```python
from build123d import *

# Parameters (mm, degrees)
CROQUIS2_W              = 20
CROQUIS2_H              = 10
SALIENTE_EXTRUIR1_DEPTH = 3
SALIENTE_EXTRUIR2_DEPTH = 2
CROQUIS4_W              = 3.2
CROQUIS4_H              = 5.473345926
CORTAR_EXTRUIR1_DEPTH   = 4
CROQUIS5_R              = 2.25
SALIENTE_EXTRUIR3_DEPTH = 3.2
CROQUIS6_R              = 1.5
CORTAR_EXTRUIR2_DEPTH   = 24.003733896
CROQUIS7_W              = 0.6
CROQUIS7_H              = 4.5
SALIENTE_EXTRUIR4_DEPTH = 1.75
CROQUIS8_R              = 0.9
CORTAR_EXTRUIR3_DEPTH   = 28.017462518


with BuildPart() as part:
    # Croquis2 → Saliente-Extruir1 (new, symmetric)
    with BuildSketch(Plane(origin=(0, 0, 0), x_dir=(0, 0, -1), z_dir=(1, 0, 0))):
        Rectangle(CROQUIS2_W, CROQUIS2_H)
    extrude(amount=SALIENTE_EXTRUIR1_DEPTH, both=True)

    # Croquis3 → Saliente-Extruir2 (add, symmetric)
    with BuildSketch(Plane(origin=(0, 0, 0), x_dir=(0, 0, -1), z_dir=(1, 0, 0))):
        with BuildLine():
            Line((-4.3, 5), (-4.3, 6.3))
            ThreePointArc((-4.3, 6.3), (-4.153553391, 6.653553391), (-3.8, 6.8))
            Line((-3.8, 6.8), (-2.5, 6.8))
            ThreePointArc((-2.5, 6.8), (-2.146446609, 6.653553391), (-2, 6.3))
            Line((-2, 6.3), (-2, 5))
            Line((-2, 5), (-4.3, 5))
        make_face()
        with BuildLine():
            Line((-7.25, 5), (-7.559492191, 6.592199292))
            Line((-7.559492191, 6.592199292), (6.919218672, 13.724276953))
            Line((6.919218672, 13.724276953), (5.46098718, 16.68460817))
            ThreePointArc((5.46098718, 16.68460817), (6.257555216, 19.027785364), (8.60073241, 18.231217328))
            Line((8.60073241, 18.231217328), (10.235719234, 14.912058085))
            Line((10.235719234, 14.912058085), (-6.654286119, 6.592199292))
            Line((-6.654286119, 6.592199292), (-7.115345765, 6.365085619))
            Line((-7.115345765, 6.365085619), (-6.85, 5))
            Line((-6.85, 5), (-7.25, 5))
        make_face()
    extrude(amount=SALIENTE_EXTRUIR2_DEPTH, both=True)

    # Croquis4 → Cortar-Extruir1 (cut)
    with BuildSketch(Plane(origin=(0, 5.422686469, -11.008504563), x_dir=(1, 0, 0), z_dir=(0, -0.4418883309364162, 0.8970700658155017))):
        with Locations((0, 11.990789002)):
            Rectangle(CROQUIS4_W, CROQUIS4_H)
    extrude(amount=-CORTAR_EXTRUIR1_DEPTH, mode=Mode.SUBTRACT)

    # Croquis5 → Saliente-Extruir3 (add)
    with BuildSketch(Plane.ZY.offset(-1.6)):
        with Locations(Location((-7.030859795, 17.457912749, 0), (0, 0, 192.71801499))):
            Circle(CROQUIS5_R)
    extrude(amount=SALIENTE_EXTRUIR3_DEPTH)

    # Croquis6 → Cortar-Extruir2 (cut, through all)
    with BuildSketch(Plane(origin=(3, 0, 0), x_dir=(0, 0, -1), z_dir=(1, 0, 0))):
        with Locations((-6, -2.5)):
            Circle(CROQUIS6_R)
        with Locations((3.5, -2.5)):
            Circle(CROQUIS6_R)
    extrude(amount=-CORTAR_EXTRUIR2_DEPTH, mode=Mode.SUBTRACT)

    # Croquis7 → Saliente-Extruir4 (add, symmetric)
    with BuildSketch(Plane(origin=(0, 0, 0), x_dir=(0, 0, -1), z_dir=(1, 0, 0))):
        with Locations((-7.7, -7.25)):
            Rectangle(CROQUIS7_W, CROQUIS7_H)
        with Locations((1.3, -7.25)):
            Rectangle(CROQUIS7_W, CROQUIS7_H)
        with Locations((8.3, -7.25)):
            Rectangle(CROQUIS7_W, CROQUIS7_H)
    extrude(amount=SALIENTE_EXTRUIR4_DEPTH, both=True)

    # Croquis8 → Cortar-Extruir3 (cut, through all)
    with BuildSketch(Plane.XY.offset(8)):
        with Locations(Location((0, -8.2, 0), (0, 0, 270))):
            Circle(CROQUIS8_R)
        Polygon((-1.75, -9), (-1.25, -9.5), (-1.75, -9.5), align=None)
        Polygon((1.25, -9.5), (1.75, -9), (1.75, -9.5), align=None)
    extrude(amount=-CORTAR_EXTRUIR3_DEPTH, mode=Mode.SUBTRACT)


solid = part.part
```
Design review of the part built by this model. Coordinates are the model's own, in mm. A direction names the side the tool comes from. Coordinates: 2 decimals unless noted, no trailing zeros. Loops run counter-clockwise (first coordinate to the right, second up) from the corner with the lowest first, then second, coordinate; pieces in that order, holes last. Notation, with made-up numbers: (84.25, -31) - (113.25, -31) arc R19 cw to (113.25, -11) - close; hole circle Ø8 at (-30.75, 25). An arc over 180 degrees is marked (long way). Use CSV: the item, a comma, the result in double quotes. Start each with the question number.
1) Consider section A-A on y = -8.2. Write out the cut boundary in (x, z).
2) Consider section C-C on y = -2.5. Write out the cut boundary in (x, z).
3) The part is to be moulded in two halves that separate along X. For faces 1 (the flat face through (0, -7, -8)), 2 (the flat face through (3, 0, 0)), 3 (the flat face through (-1.6, 15, -8)), say which applies: +X half, -X half, draft (parallel to the pull), parting line (faces both ways), or undercut.
4) Wall thickness on L1, parallel to X at y = -8.2, z = -8.5; L2, parallel to Y at x = -0.1, z = 6.5; L3, parallel to Z at x = 2.35, y = 3.75: over which ranges is each line inside the solid? List them lowest first. Write a range as from..to.
5) For pin 1 Ø1 at (x, z) = (0.5, 6) entering from +Y; pin 2 Ø1.6 at (x, y) = (0, -8.2) entering from +Z; pin 3 Ø1 at (x, z) = (-1, 3.5) entering from +Y; pin 4 Ø1.8 at (x, y) = (0, -7.5) entering from +Z, all flat-tipped, find the tip position at first contact; note any pin that passes through.
6) Consider section D-D on z = 6. Write out the cut boundary in (x, y), then the cut area to 3 significant figures.
7) Tool access review of faces 4 (the flat face through (1.8, 15.18, -6.2)), 5 (the flat face through (-2, 13, -6)), 6 (the flat face through (0, -7, -1)): name each direction out of +Z, -Z, +X, -X, +Y, -Y from which nothing blocks a thin tool from reaching the whole face with its end or side.
8) Consider section B-B on x = 2.3. Write out the cut boundary in (y, z).
Geometry says:
1,outline,"(-1.75, -8.6) - (-0.9, -8.6) - (-0.9, -8) - (-1.75, -8) - close; (-1.75, -1.6) - (-0.9, -1.6) - (-0.9, -1) - (-1.75, -1) - close; (-1.75, 7.4) - (-0.9, 7.4) - (-0.9, 8) - (-1.75, 8) - close; (0.9, -8.6) - (1.75, -8.6) - (1.75, -8) - (0.9, -8) - close; (0.9, -1.6) - (1.75, -1.6) - (1.75, -1) - (0.9, -1) - close; (0.9, 7.4) - (1.75, 7.4) - (1.75, 8) - (0.9, 8) - close"
2,outline,"(-3, -10) - (3, -10) - (3, -5) - (-3, -5) - close; (-3, -2) - (3, -2) - (3, 4.5) - (-3, 4.5) - close; (-3, 7.5) - (3, 7.5) - (3, 10) - (-3, 10) - close"
3,face 1,"draft"
3,face 2,"+X half"
3,face 3,"undercut"
4,L1,"-1.75..-0.9, 0.9..1.75"
4,L2,"-5..-3.91, -1.09..5, 6.67..7.11"
4,L3,"-10..10"
5,pin 1,"y = 7.61"
5,pin 2,"through"
5,pin 3,"y = 8.84"
5,pin 4,"z = 8"
6,outline,"(-3, -5) - (3, -5) - (3, -4) - (-3, -4) - close; (-3, -1) - (3, -1) - (3, 5) - (-3, 5) - close; (-2, 6.91) - (2, 6.91) - (2, 7.36) - (-2, 7.36) - close"
6,area,"43.8 mm^2"
7,face 4,"+Z, +X"
7,face 5,"+Z, -Z, -X, +Y"
7,face 6,"+X, -X, -Y"
8,outline,"(-5, -10) - (5, -10) - (5, 10) - (-5, 10) - close; hole circle Ø3 at (-2.5, -3.5); hole circle Ø3 at (-2.5, 6)"
